```python
from build123d import *

# Parameters (mm, degrees)
SKETCH1_R           = 10
SKETCH1_R_2         = 12.5
SKETCH1_R_3         = 15
SKETCH1_R_4         = 17.5
SKETCH1_R_5         = 20
SKETCH1_RX          = 32.743853127
SKETCH1_RY          = 15.28219651
SKETCH1_RX_2        = 19.895942638
SKETCH1_RY_2        = 7.410554201
SKETCH1_RX_3        = 13.340096181
SKETCH1_RY_3        = 3.178438996
BOSS_EXTRUDE1_DEPTH = 2
CHAMFER1_SIZE       = 1.2


with BuildPart() as part:
    # Sketch1 → Boss-Extrude1 (new body)
    with BuildSketch(Plane(origin=(0, 0, 0), x_dir=(1, 0, 0), z_dir=(0, 1, 0))):
        with BuildLine():
            Line((104.360328165, 41.874385695), (-44.558327228, 41.874385695))
            ThreePointArc((-44.558327228, 41.874385695), (-51.62939504, 38.945453507), (-54.558327228, 31.874385695))
            Line((-54.558327228, 31.874385695), (-54.558327228, -24.473029172))
            ThreePointArc((-54.558327228, -24.473029172), (-51.62939504, -31.544096984), (-44.558327228, -34.473029172))
            Line((-44.558327228, -34.473029172), (104.360328165, -34.473029172))
            ThreePointArc((104.360328165, -34.473029172), (111.431395977, -31.544096984), (114.360328165, -24.473029172))
            Line((114.360328165, -24.473029172), (114.360328165, 31.874385695))
            ThreePointArc((114.360328165, 31.874385695), (111.431395977, 38.945453507), (104.360328165, 41.874385695))
        make_face()
        with Locations(Location((-39.497024424, 17.963335967, 0), (0, 0, 270))):
            Circle(SKETCH1_R, mode=Mode.SUBTRACT)
        with Locations(Location((-14.497024424, 17.963335967, 0), (0, 0, 270))):
            Circle(SKETCH1_R_2, mode=Mode.SUBTRACT)
        with Locations(Location((15.502975576, 17.963335967, 0), (0, 0, 270))):
            Circle(SKETCH1_R_3, mode=Mode.SUBTRACT)
        with Locations(Location((50.502975576, 17.963335967, 0), (0, 0, 270))):
            Circle(SKETCH1_R_4, mode=Mode.SUBTRACT)
        with Locations(Location((90.502975576, 17.963335967, 0), (0, 0, 270))):
            Circle(SKETCH1_R_5, mode=Mode.SUBTRACT)
        with Locations(Location((-15.967241465, -13.751099436), (0, 0, -1.014060982))):
            Ellipse(SKETCH1_RX, SKETCH1_RY, mode=Mode.SUBTRACT)
        with Locations(Location((42.696291751, -14.330592911), (0, 0, 0))):
            Ellipse(SKETCH1_RX_2, SKETCH1_RY_2, mode=Mode.SUBTRACT)
        with Locations(Location((83.377613056, -14.330592911), (0, 0, 180))):
            Ellipse(SKETCH1_RX_3, SKETCH1_RY_3, mode=Mode.SUBTRACT)
    extrude(amount=BOSS_EXTRUDE1_DEPTH)

    # Chamfer1
    chamfer1_edges = [part.edges().sort_by_distance(p)[0] for p in [
        (-39.497024424, 2, -27.963335967),
        (-14.497024424, 2, -30.463335967),
        (15.502975576, 2, -32.963335967),
        (50.502975576, 2, -35.463335967),
        (90.502975576, 2, -37.963335967),
        (-48.707079481, 2, 13.305388474),
        (96.685374341, 2, 14.109425159),
        (22.804693335, 2, 14.485444524),
    ]]
    chamfer(chamfer1_edges, length=CHAMFER1_SIZE)


solid = part.part
```
Verification items for the finished model (mm, model axes). Give positions to 0.01 mm unless a question says otherwise; leave off trailing zeros. Answer as CSV lines item,"result". Start each with the question number.
Item 1: Gauge pin test, flat end, axial feed: pin 1 (8 mm diameter, centred on x = -14.5, z = 3, fed in from -Y) (3 decimals). Record the tip position at first contact, or that the pin passes through.
Item 2: Material ranges on L1, parallel to Z at x = 91.5, y = 1.75; L2, parallel to Z at x = 13, y = 0.65; L3, parallel to X at y = 1.05, z = -9 (3 decimals), recorded low to high.
Item 3: Section check A-A, the plane x = 40.5. State how many separate pieces and enclosed holes the cut face has, plus the area to 3 significant figures.
Item 4: Mould release check, pull along Z, two halves, no side actions. Record for faces 1 (the face through (29, 2, -4)), 2 (the face through (-6.05, 0.39, -27.18)), 3 (the face through (-51.707, 0.986, 31.466)): released by +Z, released by -Z, zero draft, split by the parting line, or undercut.
Filled in:
1,pin 1,"through"
2,L1,"-41.87 to -38.89, 2.96 to 10.84, 17.82 to 34.47"
2,L2,"-41.87 to -32.75, -3.17 to 7.03, 21.27 to 34.47"
2,L3,"-54.558 to -44.469, -34.525 to -23.565, -5.429 to 3.165, 27.841 to 35.182, 65.824 to 72.345, 108.661 to 114.36"
3,separate pieces,"3"
3,enclosed holes,"0"
3,area,"62.6 mm^2"
4,face 1,"zero draft"
4,face 2,"undercut"
4,face 3,"released by +Z"
